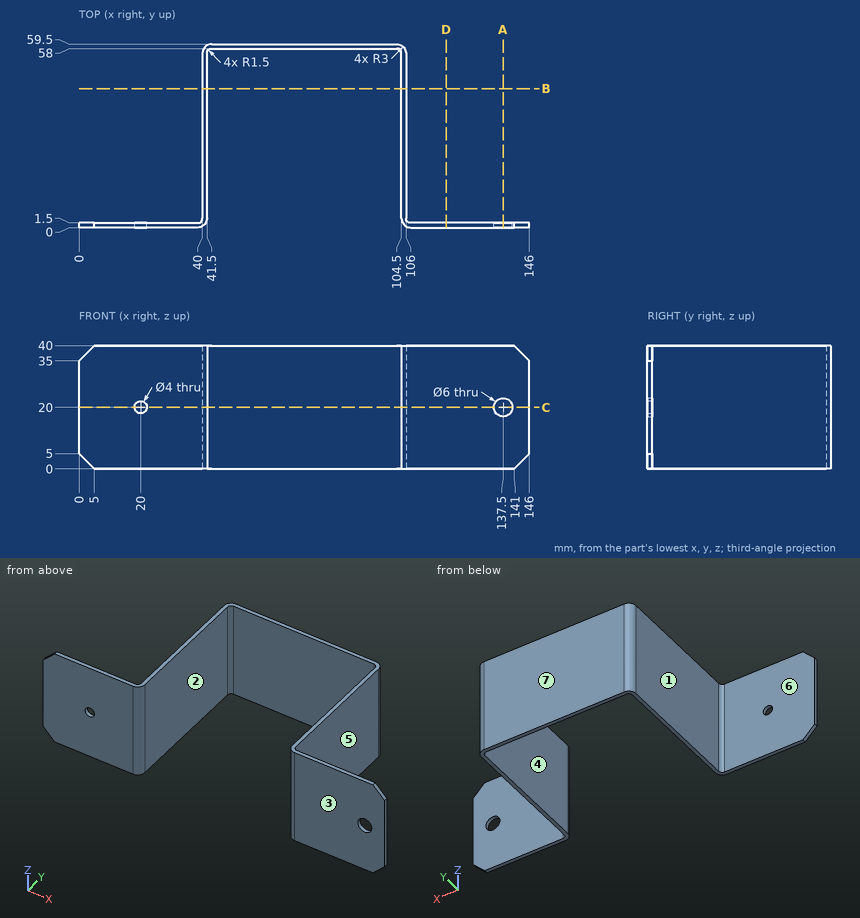
Study the drawing (mm; zero at the part's minimum x, y, z) and answer. A direction names the side the tool comes from. Coordinates: 2 decimals unless noted, no trailing zeros. Loops run counter-clockwise (first coordinate to the right, second up) from the corner with the lowest first, then second, coordinate; pieces in that order, holes last. Notation, with made-up numbers: (61, 73) -> (79, 73) arc R38 cw to (79, 112) -> close; hole circle Ø11 at (64, -6.5). An arc over 180 degrees is marked (long way). Answer in a Markdown table with one row per item. Add a question column.
1. For the marked faces 4, 5, 6 and 7, determine the directions among +Z, -Z, +X, -X, +Y, -Y from which every point of the face is accessible in a straight line to the end or side of a thin tool.
2. Determine the mould class of the marked faces 1, 2 and 3 for opening direction X: +X half, -X half, draft (parallel to the pull), parting line (faces both ways), or undercut.
3. The part is cut by section D-D, the plane x = 119. Write down the section's boundary in (y, z), then the cut area to 3 significant figures.
4. The part is cut by section C-C, the plane z = 20. Write down the section's boundary in (x, y), then the cut area to 3 significant figures.
5. The part is cut by section B-B, the plane y = 45. Write down the section's boundary in (x, z).
6. The part is cut by section A-A, the plane x = 137.5. Write down the section's boundary in (y, z), then the cut area to 3 significant figures.
7. Flat-ended cylindrical pins translate along their axes: P1, Ø20, axis at y = 34.5, z = 12.5, coming from the -X side; P2, Ø6, axis at x = 36.5, y = 43, coming from the +Z side; P3, Ø8, axis at x = 81, z = 22, coming from the -Y side; P4, Ø1.5, axis at y = 42.5, z = 8.5, coming from the +X side. Find the tip coordinate at first contact, or state that the pin passes through.
8. Consider line 1 (X direction, y = 19.5, z = 15); line 2 (Z direction, x = 137.5, y = 0.35); line 3 (Y direction, x = 127, z = 35). Determine where each line is inside the solid, lowest interval first. Write a range as [from, to].
Answer below:
| question | item | result |
|---|---|---|
| 1 | face 4 | +Z, -Z, -Y |
| 1 | face 5 | +Z, -Z, +X, +Y |
| 1 | face 6 | +Z, -Z, -X, +Y |
| 1 | face 7 | +Z, -Z, +X, -X, +Y |
| 2 | face 1 | -X half |
| 2 | face 2 | undercut |
| 2 | face 3 | draft |
| 3 | outline | (0, 0) -> (1.5, 0) -> (1.5, 40) -> (0, 40) -> close |
| 3 | area | 60.0 mm2 |
| 4 | outline | (0, 0) -> (18, 0) -> (18, 1.5) -> (0, 1.5) -> close; (22, 0) -> (38.5, 0) arc R3 ccw to (41.5, 3) -> (41.5, 56.5) arc R1.5 cw to (43, 58) -> (103, 58) arc R1.5 cw to (104.5, 56.5) -> (104.5, 3) arc R3 ccw to (107.5, 0) -> (134.5, 0) -> (134.5, 1.5) -> (107.5, 1.5) arc R1.5 cw to (106, 3) -> (106, 56.5) arc R3 ccw to (103, 59.5) -> (43, 59.5) arc R3 ccw to (40, 56.5) -> (40, 3) arc R1.5 cw to (38.5, 1.5) -> (22, 1.5) -> close; (140.5, 0) -> (146, 0) -> (146, 1.5) -> (140.5, 1.5) -> close |
| 4 | area | 372 mm2 |
| 5 | outline | (40, 0) -> (41.5, 0) -> (41.5, 40) -> (40, 40) -> close; (104.5, 0) -> (106, 0) -> (106, 40) -> (104.5, 40) -> close |
| 6 | outline | (0, 0) -> (1.5, 0) -> (1.5, 17) -> (0, 17) -> close; (0, 23) -> (1.5, 23) -> (1.5, 40) -> (0, 40) -> close |
| 6 | area | 51.0 mm2 |
| 7 | P1 | x = 40 |
| 7 | P2 | through |
| 7 | P3 | y = 58 |
| 7 | P4 | x = 106 |
| 8 | line 1 | [40, 41.5], [104.5, 106] |
| 8 | line 2 | [0, 17], [23, 40] |
| 8 | line 3 | [0, 1.5] |
